Check sheet for the modelled part. Datum: model origin and axes. Units: mm. A direction names the side the tool comes from. Give positions to 0.01 mm unless a question says otherwise; leave off trailing zeros. Order: outer loops, then holes, each group sorted by start corner. A loop starts at its lowest first (then second) coordinate and runs counter-clockwise, first axis right, second up. Notation, with made-up numbers: (38, 37) - (84, 37) arc R14 ccw to (84, 57) - close; hole circle Ø9 at (-12.5, -28). An arc over 180 degrees is marked (long way). Answer in a Markdown table with one row per item.
from build123d import *

# Parameters (mm, degrees)
ESQUISSE1_R             = 8.3
BOSS_EXTRU_1_DEPTH      = 10.5
BOSS_EXTRU_1_TAPER      = 10
ESQUISSE2_R             = 4
ENL_V_MAT_EXTRU_1_DEPTH = 2
ESQUISSE3_R             = 2
ENL_V_MAT_EXTRU_2_DEPTH = 14
CONG_1_R                = 1


with BuildPart() as part:
    # Esquisse1 → Boss.-Extru.1 (new body)
    with BuildSketch(Plane.XY):
        Circle(ESQUISSE1_R)
    extrude(amount=BOSS_EXTRU_1_DEPTH, taper=BOSS_EXTRU_1_TAPER)

    # Esquisse2 → Enlèv. mat.-Extru.1 (cut)
    with BuildSketch(Plane.XY.offset(10.5)):
        Circle(ESQUISSE2_R)
    extrude(amount=-ENL_V_MAT_EXTRU_1_DEPTH, mode=Mode.SUBTRACT)

    # Esquisse3 → Enlèv. mat.-Extru.2 (cut)
    with BuildSketch(Plane.XY.offset(8.5)):
        Circle(ESQUISSE3_R)
    extrude(amount=-ENL_V_MAT_EXTRU_2_DEPTH, mode=Mode.SUBTRACT)

    # Congé1
    cong_1_edges = [part.edges().sort_by_distance(p)[0] for p in [
        (-6.448566703, 0, 10.5),
    ]]
    fillet(cong_1_edges, radius=CONG_1_R)


solid = part.part
(1) Thickness scan on L1, parallel to Y at x = 0, z = 9.85; L2, parallel to Y at x = 0, z = 5.5; L3, parallel to Z at x = 3.75, y = -4.25. Record the ranges inside material, lowest first.
Geometry says:
| item | result |
|---|---|
| L1 | -6.55 to -4, 4 to 6.55 |
| L2 | -7.33 to -2, 2 to 7.33 |
| L3 | 0 to 10.5 |
(2) Mould release check, pull along X, two halves, no side actions. Record for faces 3 (the conical face through (6.9, 2.2, 6)), 4 (the cylindrical face through (0, -2, 4)), 5 (the flat face through (2, -4, 10.5)): pulls with the +X half, pulls with the -X half, needs draft (parallel to the pull), parting line crosses it, or undercut.
Geometry says:
| item | result |
|---|---|
| face 3 | parting line crosses it |
| face 4 | undercut |
| face 5 | needs draft |
(3) Gauge pin test, flat ends, axial feed: P1, Ø5, axis at x = -4, z = 9, coming from the +Y side; P2, Ø4, axis at x = 1.5, y = -1, coming from the +Z side; P3, Ø3, axis at x = 4.5, z = 3, coming from the -Y side. Record the tip position at first contact, or that the pin passes through.
Geometry says:
| item | result |
|---|---|
| P1 | y = 6.69 |
| P2 | z = 8.5 |
| P3 | y = -7.23 |
(4) Access from +Z, -Z, +X, -X, +Y, -Y to the whole of each face (thin tool, end or side, straight path). Record for faces 1 (the flat face through (-2, -1, 8.5)), 2 (the flat face through (2, -2, 0)).
Geometry says:
| item | result |
|---|---|
| face 1 | +Z |
| face 2 | -Z, +X, -X, +Y, -Y |
(5) Cross-section at C-C, the plane z = 9.25. Record the cut outline in (x, y), then the cut area to 3 significant figures.
Geometry says:
| item | result |
|---|---|
| outline | circle Ø13.34 at (0, 0); hole circle Ø8 at (0, 0) |
| area | 89.5 mm² |
(6) Cross-section at A-A, the plane x = 0. Record the cut outline in (y, z).
Geometry says:
| item | result |
|---|---|
| outline | (-8.3, 0) - (-2, 0) - (-2, 8.5) - (-4, 8.5) - (-4, 10.5) - (-5.61, 10.5) arc R1 ccw to (-6.59, 9.67) - close; (2, 0) - (8.3, 0) - (6.59, 9.67) arc R1 ccw to (5.61, 10.5) - (4, 10.5) - (4, 8.5) - (2, 8.5) - close |
(7) Cross-section at D-D, the plane z = 7.25. Record the cut outline in (x, y).
Geometry says:
| item | result |
|---|---|
| outline | circle Ø14.04 at (0, 0); hole circle Ø4 at (0, 0) |
